Geometry check sheet. Reference: the model listing, model coordinates, mm. Face numbers are marked on the shaded views. A direction names the side the tool comes from. Give positions to 0.01 mm unless a question says otherwise; leave off trailing zeros. Write each loop counter-clockwise with the first axis right and the second up, starting at its lowest first coordinate (ties: lowest second). Pieces come first, ordered by that corner, then holes.
(1) Mould release check, pull along X, two halves, no side actions. Record for the marked faces 1, 2 and 3: +X half, -X half, draft (parallel to the pull), parting line (faces both ways), or undercut.
(2) Cross-section at B-B (x = 0). Record the boundary of the cut face in (y, z).
(3) Thickness scan on line 1 along X through (y, z) = (4, 0); line 2 along X through (y, z) = (22, 0); line 3 along X through (y, z) = (3.5, -2). Record the ranges inside material, lowest first.
(4) Depth check by flat-ended pin: P1, Ø12, axis at x = 31.5, y = 6.5, coming from the +Z side; P2, Ø6, axis at y = 11, z = -9, coming from the -X side; P3, Ø2, axis at x = 35.5, z = 23, coming from the -Y side; P4, Ø6, axis at x = -34, z = 25.5, coming from the +Y side. Enter the tip coordinate at first touch or a pass-through.
(5) Cross-section at A-A (z = -40). Record the boundary of the cut face in (x, y), and give its area (3 significant figures).
(6) Cross-section at C-C (x = 40). Record the boundary of the cut face in (y, z).
(7) Cross-section at D-D (z = 0). Record the boundary of the cut face in (x, y), and give its area (3 significant figures).
(8) Tool access check on the marked faces 4 and 5. Record the directions out of +Z, -Z, +X, -X, +Y, -Y that give a thin tool (end or side, any length) a straight path to the whole face; none if there is none.
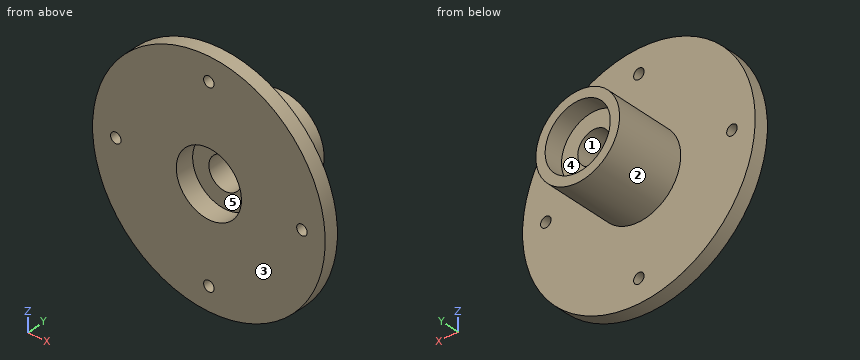
```python
from build123d import *

# Parameters (mm, degrees)
SKETCH2_R           = 50
BOSS_EXTRUDE1_DEPTH = 6
SKETCH3_R           = 18
BOSS_EXTRUDE2_DEPTH = 30
SKETCH4_R           = 7
CUT_EXTRUDE1_DEPTH  = 80.3473377
SKETCH5_R           = 14
CUT_EXTRUDE2_DEPTH  = 8
CUT_EXTRUDE3_START  = -8
SKETCH6_R           = 14
CUT_EXTRUDE3_DEPTH  = 8
SKETCH7_R           = 2.25
CUT_EXTRUDE4_DEPTH  = 80.3473377
CIRPATTERN1_COUNT   = 4


with BuildPart() as part:
    # Sketch2 → Boss-Extrude1 (new body)
    with BuildSketch(Plane(origin=(0, 0, 0), x_dir=(1, 0, 0), z_dir=(0, 1, 0))):
        with Locations(Location((0, 0, 0), (0, 0, 270))):
            Circle(SKETCH2_R)
    extrude(amount=BOSS_EXTRUDE1_DEPTH)

    # Sketch3 → Boss-Extrude2 (add)
    with BuildSketch(Plane(origin=(0, 6, 0), x_dir=(1, 0, 0), z_dir=(0, 1, 0))):
        with Locations(Location((0, 0, 0), (0, 0, 270))):
            Circle(SKETCH3_R)
    extrude(amount=BOSS_EXTRUDE2_DEPTH)

    # Sketch4 → Cut-Extrude1 (cut, through all)
    with BuildSketch(Plane(origin=(0, 36, 0), x_dir=(1, 0, 0), z_dir=(0, 1, 0))):
        with Locations(Location((0, 0, 0), (0, 0, 270))):
            Circle(SKETCH4_R)
    extrude(amount=-CUT_EXTRUDE1_DEPTH, mode=Mode.SUBTRACT)

    # Sketch5 → Cut-Extrude2 (cut)
    with BuildSketch(Plane(origin=(0, 36, 0), x_dir=(1, 0, 0), z_dir=(0, 1, 0))):
        with Locations(Location((0, 0, 0), (0, 0, 270))):
            Circle(SKETCH5_R)
    extrude(amount=-CUT_EXTRUDE2_DEPTH, mode=Mode.SUBTRACT)

    # Sketch6 → Cut-Extrude3 (cut)
    with BuildSketch(Plane.XZ.offset(CUT_EXTRUDE3_START)):
        with Locations(Location((0, 0, 0), (0, 0, 90))):
            Circle(SKETCH6_R)
    extrude(amount=CUT_EXTRUDE3_DEPTH, mode=Mode.SUBTRACT)

    # Sketch7 → Cut-Extrude4 (cut, through all)
    with BuildSketch(Plane.XZ):
        with Locations(Location((40, 0, 0), (0, 0, 270))):
            Circle(SKETCH7_R)
    cut_extrude4 = extrude(amount=-CUT_EXTRUDE4_DEPTH, mode=Mode.SUBTRACT)

    # CirPattern1: Cut-Extrude4 ×4 about axis
    cirpattern1_axis = Axis((0, 0, 0), (0, 1, 0))
    for i in range(1, CIRPATTERN1_COUNT):
        add(cut_extrude4.rotate(cirpattern1_axis, i * 360 / CIRPATTERN1_COUNT), mode=Mode.SUBTRACT)


solid = part.part
```
Reply:
1. face 1: undercut
1. face 2: parting line
1. face 3: draft
2. outline: (0, -50) - (6, -50) - (6, -42.25) - (0, -42.25) - close; (0, -37.75) - (6, -37.75) - (6, -18) - (36, -18) - (36, -14) - (28, -14) - (28, -7) - (8, -7) - (8, -14) - (0, -14) - close; (0, 14) - (8, 14) - (8, 7) - (28, 7) - (28, 14) - (36, 14) - (36, 18) - (6, 18) - (6, 37.75) - (0, 37.75) - close; (0, 42.25) - (6, 42.25) - (6, 50) - (0, 50) - close
3. line 1: x = -50 to -42.25, -37.75 to -14, 14 to 37.75, 42.25 to 50
3. line 2: x = -18 to -7, 7 to 18
3. line 3: x = -49.96 to -41.03, -38.97 to -13.86, 13.86 to 38.97, 41.03 to 49.96
4. P1: stops at z = 43
4. P2: stops at x = -16.97
4. P3: stops at y = 0
4. P4: stops at y = 6
5. outline: (-30, 0) - (-2.25, 0) - (-2.25, 6) - (-30, 6) - close; (2.25, 0) - (30, 0) - (30, 6) - (2.25, 6) - close
5. area: 333 mm2
6. outline: (0, -30) - (6, -30) - (6, -2.25) - (0, -2.25) - close; (0, 2.25) - (6, 2.25) - (6, 30) - (0, 30) - close
7. outline: (-50, 0) - (-42.25, 0) - (-42.25, 6) - (-50, 6) - close; (-37.75, 0) - (-14, 0) - (-14, 8) - (-7, 8) - (-7, 28) - (-14, 28) - (-14, 36) - (-18, 36) - (-18, 6) - (-37.75, 6) - close; (7, 8) - (14, 8) - (14, 0) - (37.75, 0) - (37.75, 6) - (18, 6) - (18, 36) - (14, 36) - (14, 28) - (7, 28) - close; (42.25, 0) - (50, 0) - (50, 6) - (42.25, 6) - close
7. area: 898 mm2
8. face 4: +Y
8. face 5: -Y
